```python
from build123d import *

# Parameters (mm, degrees)
F0_W      = 100
F0_H      = 40
F1_DEPTH  = 2
F2_SIZE   = 1.99999
F3_W      = 84
F3_H      = 24
F4_DEPTH  = 5
F5_R      = 1.5
F6_DEPTH  = 2.001
F7_R      = 5
F8_R      = 10
F9_DEPTH  = 7.001
F11_DEPTH = 7.001
F13_DEPTH = 7.001
F15_DEPTH = 1.5
F17_DEPTH = 1.5
F19_DEPTH = 1.5


# Not quite as in the source:
# - a fillet or chamfer is up to 0.001 mm smaller than in the source, because OpenCascade refuses the exact size


with BuildPart() as f1:
    # F0 (on Front) → F1 (new body)
    with BuildSketch(Plane.XZ):
        with Locations((50, 20)):
            Rectangle(F0_W, F0_H)
    extrude(amount=F1_DEPTH)

    # F2 (size 2 in the source; OpenCascade refuses exactly that, so slightly less here)
    f2_edges = [f1.edges().sort_by_distance(p)[0] for p in [
        (100, -2, 20),
        (50, -2, 40),
        (50, -2, 0),
        (0, -2, 20),
    ]]
    chamfer(f2_edges, length=F2_SIZE)

    # F3 (on face) → F4 (join)
    with BuildSketch(Plane(origin=(0, 0, 0), x_dir=(-1, 0, 0), z_dir=(0, 1, 0))):
        with Locations((-50, 20)):
            Rectangle(F3_W, F3_H)
    extrude(amount=F4_DEPTH)

    # F5 (on face) → F6 (cut, through all)
    with BuildSketch(Plane(origin=(0, 0, 0), x_dir=(-1, 0, 0), z_dir=(0, 1, 0))):
        with Locations((-94.5, 34.5)):
            Circle(F5_R)
        with Locations((-94.5, 5.5)):
            Circle(F5_R)
        with Locations((-5.5, 34.5)):
            Circle(F5_R)
        with Locations((-5.5, 5.5)):
            Circle(F5_R)
    extrude(amount=-F6_DEPTH, mode=Mode.SUBTRACT)

    # F7
    f7_edges = [f1.edges().sort_by_distance(p)[0] for p in [
        (92, 2.5, 8),
        (92, 2.5, 32),
        (8, 2.5, 8),
        (8, 2.5, 32),
    ]]
    fillet(f7_edges, radius=F7_R)

    # F8 (on face) → F9 (cut, through all)
    with BuildSketch(Plane(origin=(0, 5, 0), x_dir=(-1, 0, 0), z_dir=(0, 1, 0))):
        with Locations((-80, 20)):
            Circle(F8_R)
        with Locations((-55, 20)):
            Circle(F8_R)
        with Locations((-20, 20)):
            Circle(F8_R)
    extrude(amount=-F9_DEPTH, mode=Mode.SUBTRACT)

    # F10 (on face) → F11 (cut, through all)
    with BuildSketch(Plane(origin=(0, 5, 0), x_dir=(-1, 0, 0), z_dir=(0, 1, 0))):
        with BuildLine():
            Line((-89.9215674165, 21.25), (-91, 21.25))
            Line((-91, 21.25), (-91, 18.75))
            Line((-91, 18.75), (-89.9215674165, 18.75))
            ThreePointArc((-89.9215674165, 18.75), (-90, 20), (-89.9215674165, 21.25))
        make_face()
        with BuildLine():
            Line((-64.9215674165, 21.25), (-66, 21.25))
            Line((-66, 21.25), (-66, 18.75))
            Line((-66, 18.75), (-64.9215674165, 18.75))
            ThreePointArc((-64.9215674165, 18.75), (-65, 20), (-64.9215674165, 21.25))
        make_face()
        with BuildLine():
            Line((-29.9215674165, 21.25), (-31, 21.25))
            Line((-31, 21.25), (-31, 18.75))
            Line((-31, 18.75), (-29.9215674165, 18.75))
            ThreePointArc((-29.9215674165, 18.75), (-30, 20), (-29.9215674165, 21.25))
        make_face()
    extrude(amount=-F11_DEPTH, mode=Mode.SUBTRACT)

    # F12 (on face) → F13 (cut, through all)
    with BuildSketch(Plane(origin=(0, 5, 0), x_dir=(-1, 0, 0), z_dir=(0, 1, 0))):
        with BuildLine():
            Line((-77.75, 30.5), (-82.25, 30.5))
            Line((-82.25, 30.5), (-82.25, 29.743587635))
            ThreePointArc((-82.25, 29.743587635), (-80, 30), (-77.75, 29.743587635))
            Line((-77.75, 29.743587635), (-77.75, 30.5))
        make_face()
        with BuildLine():
            ThreePointArc((-77.75, 10.256412365), (-80, 10), (-82.25, 10.256412365))
            Line((-82.25, 10.256412365), (-82.25, 9.5))
            Line((-82.25, 9.5), (-77.75, 9.5))
            Line((-77.75, 9.5), (-77.75, 10.256412365))
        make_face()
        with BuildLine():
            ThreePointArc((-52.75, 10.256412365), (-55, 10), (-57.25, 10.256412365))
            Line((-57.25, 10.256412365), (-57.25, 9.5))
            Line((-57.25, 9.5), (-52.75, 9.5))
            Line((-52.75, 9.5), (-52.75, 10.256412365))
        make_face()
        with BuildLine():
            Line((-52.75, 30.5), (-57.25, 30.5))
            Line((-57.25, 30.5), (-57.25, 29.743587635))
            ThreePointArc((-57.25, 29.743587635), (-55, 30), (-52.75, 29.743587635))
            Line((-52.75, 29.743587635), (-52.75, 30.5))
        make_face()
        with BuildLine():
            Line((-17.75, 30.5), (-22.25, 30.5))
            Line((-22.25, 30.5), (-22.25, 29.743587635))
            ThreePointArc((-22.25, 29.743587635), (-20, 30), (-17.75, 29.743587635))
            Line((-17.75, 29.743587635), (-17.75, 30.5))
        make_face()
        with BuildLine():
            ThreePointArc((-17.75, 10.256412365), (-20, 10), (-22.25, 10.256412365))
            Line((-22.25, 10.256412365), (-22.25, 9.5))
            Line((-22.25, 9.5), (-17.75, 9.5))
            Line((-17.75, 9.5), (-17.75, 10.256412365))
        make_face()
    extrude(amount=-F13_DEPTH, mode=Mode.SUBTRACT)

    # F14 (on face) → F15 (cut)
    with BuildSketch(Plane.XZ.offset(2)):
        with BuildLine():
            ThreePointArc((22.75, 34.55), (18.5638593384, 36.8952078799), (18.75, 32.1005102572))
            Line((18.75, 32.1005102572), (18.75, 33.3252551286))
            ThreePointArc((18.75, 33.3252551286), (19.3385621722, 36.1701851746), (21.75, 34.55))
            ThreePointArc((21.75, 34.55), (21.6201851746, 33.8885621722), (21.25, 33.3252551286))
            Line((21.25, 33.3252551286), (21.25, 32.1005102572))
            ThreePointArc((21.25, 32.1005102572), (22.3452078799, 33.1138593384), (22.75, 34.55))
        make_face()
        with BuildLine():
            Line((19.5, 34.8), (19.5, 32.8729490169))
            ThreePointArc((19.5, 32.8729490169), (20, 32.8), (20.5, 32.8729490169))
            Line((20.5, 32.8729490169), (20.5, 34.8))
            Line((20.5, 34.8), (19.5, 34.8))
        make_face()
        with BuildLine():
            ThreePointArc((19.5, 31.8458365434), (19.7489517035, 31.8114831107), (20, 31.8))
            ThreePointArc((20, 31.8), (20.2510482965, 31.8114831107), (20.5, 31.8458365434))
            Line((20.5, 31.8458365434), (20.5, 32.8729490169))
            ThreePointArc((20.5, 32.8729490169), (20, 32.8), (19.5, 32.8729490169))
            Line((19.5, 32.8729490169), (19.5, 31.8458365434))
        make_face()
    extrude(amount=-F15_DEPTH, mode=Mode.SUBTRACT)

    # F16 (on face) → F17 (cut)
    with BuildSketch(Plane.XZ.offset(2)):
        with BuildLine():
            ThreePointArc((54.1339745962, 34.05), (54.5, 33.6839745962), (55, 33.55))
            Line((55, 33.55), (54.7113248654, 34.05))
            Line((54.7113248654, 34.05), (54.1339745962, 34.05))
        make_face()
        Polygon((54.4226497308, 34.55), (54.1339745962, 34.05), (54.7113248654, 34.05), align=None)
        with BuildLine():
            Line((54.4226497308, 34.55), (54.1339745962, 35.05))
            ThreePointArc((54.1339745962, 35.05), (54, 34.55), (54.1339745962, 34.05))
            Line((54.1339745962, 34.05), (54.4226497308, 34.55))
        make_face()
        Polygon((54.7113248654, 35.05), (54.1339745962, 35.05), (54.4226497308, 34.55), align=None)
        with BuildLine():
            Line((54.7113248654, 35.05), (55, 35.55))
            ThreePointArc((55, 35.55), (54.5, 35.4160254038), (54.1339745962, 35.05))
            Line((54.1339745962, 35.05), (54.7113248654, 35.05))
        make_face()
        Polygon((55.2886751346, 35.05), (55, 35.55), (54.7113248654, 35.05), align=None)
        Polygon((55.5773502692, 34.55), (55.2886751346, 35.05), (54.7113248654, 35.05), (54.4226497308, 34.55), (54.7113248654, 34.05), (55.2886751346, 34.05), align=None)
        Polygon((54.7113248654, 34.05), (55, 33.55), (55.2886751346, 34.05), align=None)
        with BuildLine():
            ThreePointArc((55, 33.55), (55.5, 33.6839745962), (55.8660254038, 34.05))
            Line((55.8660254038, 34.05), (55.2886751346, 34.05))
            Line((55.2886751346, 34.05), (55, 33.55))
        make_face()
        with BuildLine():
            ThreePointArc((56, 34.55), (55.9659258263, 34.8088190451), (55.8660254038, 35.05))
            Line((55.8660254038, 35.05), (55.5773502692, 34.55))
            Line((55.5773502692, 34.55), (55.8660254038, 34.05))
            ThreePointArc((55.8660254038, 34.05), (55.9659258263, 34.2911809549), (56, 34.55))
        make_face()
        Polygon((55.5773502692, 34.55), (55.8660254038, 35.05), (55.2886751346, 35.05), align=None)
        with BuildLine():
            Line((55.2886751346, 35.05), (55.8660254038, 35.05))
            ThreePointArc((55.8660254038, 35.05), (55.5, 35.4160254038), (55, 35.55))
            Line((55, 35.55), (55.2886751346, 35.05))
        make_face()
        Polygon((55.2886751346, 34.05), (55.8660254038, 34.05), (55.5773502692, 34.55), align=None)
        with BuildLine():
            ThreePointArc((53.2149055698, 32.4581257506), (53.625, 32.1684301396), (54.0809309736, 31.9581257506))
            Line((54.0809309736, 31.9581257506), (54.5944872103, 32.8476312452))
            ThreePointArc((54.5944872103, 32.8476312452), (54.125, 33.0344555434), (53.7284618065, 33.3476312452))
            Line((53.7284618065, 33.3476312452), (53.2149055698, 32.4581257506))
        make_face()
        with BuildLine():
            ThreePointArc((55.9190690264, 31.9581257506), (56.375, 32.1684301396), (56.7850944302, 32.4581257506))
            Line((56.7850944302, 32.4581257506), (56.2715381935, 33.3476312452))
            ThreePointArc((56.2715381935, 33.3476312452), (55.875, 33.0344555434), (55.4055127897, 32.8476312452))
            Line((55.4055127897, 32.8476312452), (55.9190690264, 31.9581257506))
        make_face()
        with BuildLine():
            ThreePointArc((57.7041634566, 34.05), (57.7385168893, 34.2989517035), (57.75, 34.55))
            ThreePointArc((57.75, 34.55), (57.7385168893, 34.8010482965), (57.7041634566, 35.05))
            Line((57.7041634566, 35.05), (56.6770509831, 35.05))
            ThreePointArc((56.6770509831, 35.05), (56.7316667145, 34.8026467688), (56.75, 34.55))
            ThreePointArc((56.75, 34.55), (56.7316667145, 34.2973532312), (56.6770509831, 34.05))
            Line((56.6770509831, 34.05), (57.7041634566, 34.05))
        make_face()
        with BuildLine():
            Line((56.2715381935, 35.7523687548), (56.7850944302, 36.6418742494))
            ThreePointArc((56.7850944302, 36.6418742494), (56.375, 36.9315698604), (55.9190690264, 37.1418742494))
            Line((55.9190690264, 37.1418742494), (55.4055127897, 36.2523687548))
            ThreePointArc((55.4055127897, 36.2523687548), (55.875, 36.0655444566), (56.2715381935, 35.7523687548))
        make_face()
        with BuildLine():
            Line((54.5944872103, 36.2523687548), (54.0809309736, 37.1418742494))
            ThreePointArc((54.0809309736, 37.1418742494), (53.625, 36.9315698604), (53.2149055698, 36.6418742494))
            Line((53.2149055698, 36.6418742494), (53.7284618065, 35.7523687548))
            ThreePointArc((53.7284618065, 35.7523687548), (54.125, 36.0655444566), (54.5944872103, 36.2523687548))
        make_face()
        with BuildLine():
            Line((53.3229490169, 35.05), (52.2958365434, 35.05))
            ThreePointArc((52.2958365434, 35.05), (52.25, 34.55), (52.2958365434, 34.05))
            Line((52.2958365434, 34.05), (53.3229490169, 34.05))
            ThreePointArc((53.3229490169, 34.05), (53.25, 34.55), (53.3229490169, 35.05))
        make_face()
    extrude(amount=-F17_DEPTH, mode=Mode.SUBTRACT)

    # F18 (on face) → F19 (cut)
    with BuildSketch(Plane.XZ.offset(2)):
        Polygon((77, 35.7), (84, 37), (77, 37), align=None)
        Polygon((83, 35.35), (77, 35.35), (77, 34.05), align=None)
        Polygon((77, 32.4), (82, 33.7), (77, 33.7), align=None)
    extrude(amount=-F19_DEPTH, mode=Mode.SUBTRACT)


solid = f1.part
```
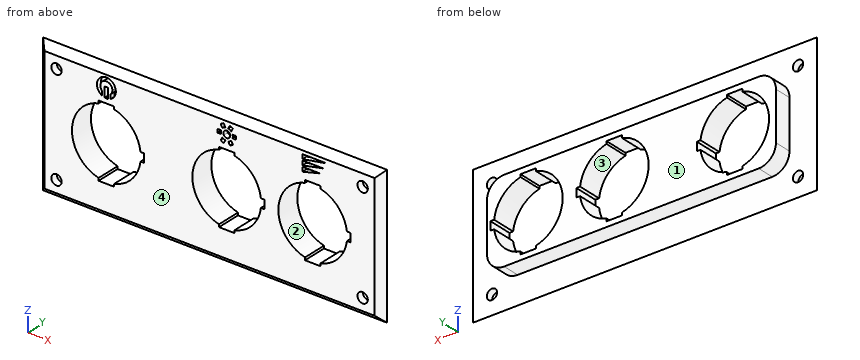
Design review of the part built by this model. Coordinates are the model's own, in mm. Face numbers are marked on the shaded views. A direction names the side the tool comes from. Round coordinates to 2 decimals unless told otherwise and drop trailing zeros. Put each result on its own line as item: value.
Q1. Consider section A-A (z = 5.5). State how many separate pieces and enclosed holes the cut face has, and give its area (3 significant figures).
Reported:
separate pieces: 3
enclosed holes: 0
area: 184 mm²
Q2. Machinability: for the marked faces 3 and 4, which of the approach directions +Z, -Z, +X, -X, +Y, -Y give a long, thin tool a straight path to every point of the face, cutting with its end or side? Answer none if there is none.
Reported:
face 3: +Y, -Y
face 4: +Z, -Z, +X, -X, -Y
Q3. To check wall thickness, follow line 1 (Z direction, x = 78, y = 1.5); line 2 (X direction, y = 2, z = 20.5); line 3 (Z direction, x = 94.5, y = -1.6). State the ranges of each line that lie inside material, in increasing order.
Reported:
line 1: 8 to 9.5, 30.5 to 32
line 2: 8 to 10.01, 31 to 45.01, 66 to 70.01, 91 to 92
line 3: 1.6 to 4, 7 to 33, 36 to 38.4
Q4. Insertion check: pin 1 Ø0.6 at (y, z) = (3, 10) entering from +X; pin 2 Ø0.5 at (x, y) = (90.5, 3) entering from +Z; pin 3 Ø1.1 at (x, y) = (57.5, -1.5) entering from -Z. Each pin has a flat end and moves straight along its axis. Give the tip position at first contact, or say it passes through.
Reported:
pin 1: x = 91.21
pin 2: z = 30.8
pin 3: z = 0.95
Q5. Draft analysis for pull direction Z (two halves, no side actions). For the marked faces 1 and 2, state which applies: released by +Z, released by -Z, zero draft, split by the parting line, or undercut.
Reported:
face 1: zero draft
face 2: undercut
